Autodesk Inventor part; units mm, degrees
ref_plane "YZ Plane" through (0, 0, 0) normal (1, 0, 0) x (0, 1, 0)
ref_plane "XZ Plane" through (0, 0, 0) normal (0, 1, 0) x (-1, 0, 0)
ref_plane "XY Plane" through (0, 0, 0) normal (0, 0, 1) x (1, 0, 0)
sketch "スケッチ1" plane through (0, 0, 0) normal (1, 0, 0) x (0, 1, 0)
  line L0 (0, 125) -> (0, -125)
  line L1 (-193.7075, 0) -> (764.5712, 0)
  arc A0 (0, 125) -> (0, -125) centre (627.6743, 0) ccw
  arc A1 (0, 125) -> (-45.1737, 25) centre (79.0119, 29.1041) ccw
  arc A2 (-45.1737, 25) -> (0, -125) centre (259.9333, 35.0832) ccw
  point P0 (0, 0)
  point P1 (0, 0)
  dimension "d0" = 250
  dimension "d1" = 640
  dimension "d16" = 100
extrude "押し出し4" add sketch "スケッチ1" along normal mid plane 950 contours A0 L1 A2 A1 | A0 A2 L1
fillet "フィレット3" radius 5 1 edges at (0, 0, 125)
fillet "フィレット3" radius 3 1 edges at (0, 0, -125)
sketch "スケッチ4" plane through (475, 0, 0) normal (1, 0, 0) x (0, 0, -1)
  circle A0 centre (23.3804, -26.1259) radius 6
  arc A1 (109.8042, -8.7665) -> (107.8747, -3.1688) centre (108.3804, -6.1259) ccw
  point P0 (0, 0)
  dimension "d21" = 12
  dimension "d22" = 85
  dimension "d23" = 20
extrude "押し出し5" cut sketch "スケッチ4" against normal through all
properties part number "styro_50_sub" material "ポリスチレン"
Input: part model. Units: mm. Frame: model coordinates. Give positions to 0.01 mm unless a question says otherwise; leave off trailing zeros. Write each loop counter-clockwise with the first axis right and the second up, starting at its lowest first coordinate (ties: lowest second). Pieces come first, ordered by that corner, then holes. Notation, with made-up numbers: (69, 55.5) -> (82, 55.5) arc R23 cw to (82, 83.5) -> close; hole circle Ø4 at (-20.5, 81.25). An arc over 180 degrees is marked (long way). Use one line per item in the form item = value. Start each with the question number.
1) Section query B-B on z = -96.5. Return the cut outline in (x, y).
2) Pin query (flat end, axial travel): pin 1 (2 mm diameter, centred on x = 123, z = -85.5, fed in from +Y); pin 2 (8 mm diameter, centred on x = -296, y = -38, fed in from +Z); pin 3 (5 mm diameter, centred on x = -136.5, y = -30.5, fed in from +Z). Return the tip coordinate at first contact, or that it passes through.
3) Ray query, probe 1 along Z at (x, y) = (59.5, -22); probe 2 along Z at (x, y) = (17.5, -13.5); probe 3 along Y at (x, z) = (369.5, 57). Return the intervals inside material, ascending. Write a range as from..to.
4) Section query A-A on z = 14. Return the cut outline in (x, y).
5) Draft query along Z for faces 1 (the flat face through (475, -24, 4)), 2 (the cylindrical face through (-6.65, -34.522, -45.463)), 3 (the cylindrical face through (-6.65, -12.326, -0.403)). Return one class per face: pulls with the +Z half, pulls with the -Z half, needs draft (parallel to the pull), parting line crosses it, or undercut.
Outcome:
q1.outline = (-475, -15.53) -> (475, -15.53) -> (475, -5.01) -> (-475, -5.01) -> close
q2.pin_1 = -6.45
q2.pin_2 = 80.75
q2.pin_3 = 92.25
q3.probe_1 = -81.99..-27.74, -19.02..101.46
q3.probe_2 = -100.66..112.05
q3.probe_3 = -42.07..-9.78
q4.outline = (-475, -44.61) -> (475, -44.61) -> (475, -12.17) -> (-475, -12.17) -> close
q5.face_1 = needs draft
q5.face_2 = pulls with the -Z half
q5.face_3 = undercut
